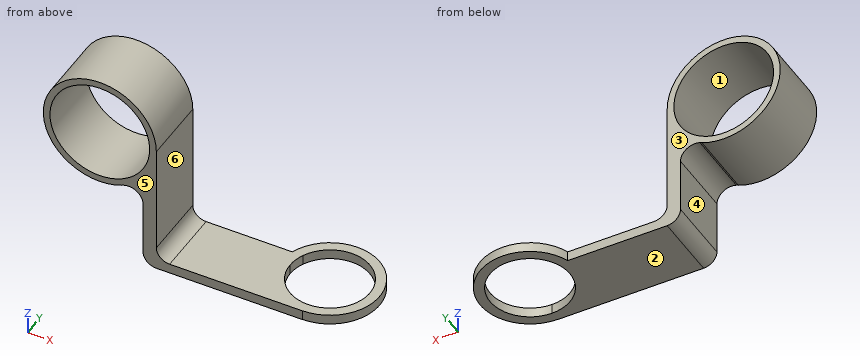
from build123d import *
from build123d.topology import SkipClean

# Parameters (mm, degrees)
SKETCH1_R           = 15
BOSS_EXTRUDE2_DEPTH = 20
CUT_EXTRUDE2_DEPTH  = 21
BOSS_EXTRUDE3_DEPTH = 3


with BuildPart() as part:
    # Sketch1 → Boss-Extrude2 (new body)
    # profile 1 of 2: a face of its own
    with BuildSketch(Plane(origin=(0, 0, 0), x_dir=(1, 0, 0), z_dir=(0, 1, 0))):
        with BuildLine():
            ThreePointArc((-50.780177481, 15.676092064), (-71.513924264, -9.412408123), (-40.357421401, 0))
            ThreePointArc((-40.357421401, 0), (-43.025497107, 9.143081868), (-50.192238582, 15.416230251))
            ThreePointArc((-50.192238582, 15.416230251), (-50.490994878, 15.535330889), (-50.780177481, 15.676092064))
        make_face()
        with Locations(Location((-57.357421401, 0, 0), (0, 0, 270))):
            Circle(SKETCH1_R, mode=Mode.SUBTRACT)
    # profile 2 of 2: a face of its own
    with BuildSketch(Plane(origin=(0, 0, 0), x_dir=(1, 0, 0), z_dir=(0, 1, 0))):
        with BuildLine():
            Line((-40.357421401, 0), (-40.357421401, 33))
            ThreePointArc((-40.357421401, 33), (-39.185848526, 35.828427125), (-36.357421401, 37))
            Line((-36.357421401, 37), (3.642578599, 37))
            Line((3.642578599, 37), (3.642578599, 40))
            Line((3.642578599, 40), (-40.357421401, 40))
            ThreePointArc((-40.357421401, 40), (-43.185848526, 38.828427125), (-44.357421401, 36))
            Line((-44.357421401, 36), (-44.357421401, 19.501688617))
            ThreePointArc((-44.357421401, 19.501688617), (-46.219952281, 15.952391985), (-50.192238582, 15.416230251))
            ThreePointArc((-50.192238582, 15.416230251), (-43.025497107, 9.143081868), (-40.357421401, 0))
        make_face()
    extrude(amount=BOSS_EXTRUDE2_DEPTH)

    # Sketch3 → Cut-Extrude2 (cut)
    with BuildSketch(Plane(origin=(0, 0, -40), x_dir=(-1, 0, 0), z_dir=(0, 0, -1))):
        with BuildLine():
            Line((-3.642578599, 20), (-3.642578599, 3))
            ThreePointArc((-3.642578599, 3), (4.842702775, 6.514718626), (8.357421401, 15))
            ThreePointArc((8.357421401, 15), (8.081425525, 17.558852734), (7.266133516, 20))
            Line((7.266133516, 20), (-3.642578599, 20))
        make_face()
        with BuildLine():
            ThreePointArc((7.266133516, 20), (-13.742083537, 21.480740698), (-3.642578599, 3))
            Line((-3.642578599, 3), (-3.642578599, 20))
            Line((-3.642578599, 20), (7.266133516, 20))
        make_face()
    extrude(amount=-CUT_EXTRUDE2_DEPTH, mode=Mode.SUBTRACT)

    # Sketch4 → Boss-Extrude3 (add)
    with SkipClean():  # the faces are left unmerged after this step: merging them gives an invalid solid
        with BuildSketch(Plane(origin=(0, 0, -40), x_dir=(-1, 0, 0), z_dir=(0, 0, -1))):
            with BuildLine():
                Line((-3.642578599, 0.051873716), (-3.642578599, 3))
                ThreePointArc((-3.642578599, 3), (-13.742083537, 21.480740698), (7.266133516, 20))
                Line((7.266133516, 20), (10.444524701, 20))
                ThreePointArc((10.444524701, 20), (-15.852965792, 23.622814157), (-3.642578599, 0.051873716))
            make_face()
        extrude(amount=-BOSS_EXTRUDE3_DEPTH)


solid = part.part
Part model, mm, in its own coordinate system. Face numbers are marked on the shaded views. A direction names the side the tool comes from. Give positions to 0.01 mm unless a question says otherwise; leave off trailing zeros. Loops run counter-clockwise (first coordinate to the right, second up) from the corner with the lowest first, then second, coordinate; pieces in that order, holes last.
(1) Pull direction Z, two halves, no side cores. Call the marked faces 1, 2 and 3: pulls with the +Z half, pulls with the -Z half, needs draft (parallel to the pull), parting line crosses it, or undercut.
Return value:
face 1: undercut
face 2: pulls with the -Z half
face 3: needs draft
(2) Band-saw the part on D-D (y = 2). Write the cut outline in (x, z), and give its area (3 significant figures).
Return value:
outline: (-50.78, -15.68) arc R4.37 cw to (-44.36, -19.5) - (-44.36, -36) arc R4 ccw to (-40.36, -40) - (11.02, -40) - (11.02, -37) - (-36.36, -37) arc R4 cw to (-40.36, -33) - (-40.36, 0) arc R17 ccw (long way) to start; hole circle Ø30 at (-57.36, 0)
area: 499 mm2
(3) Drill centre lines: line 1 along X through (y, z) = (9, -23); line 2 along Z through (x, y) = (-60, 18.25); line 3 along Z through (x, y) = (-17, 11.5). Where is each one in solid material? Low to high.
Return value:
line 1: x = -44.36 to -40.36
line 2: z = -16.79 to -14.77, 14.77 to 16.79
line 3: z = -40 to -37
(4) 3-axis set-ups, long thin cutter, end or side, ignore diameter. For the marked faces 4, 5 and 6: which of +Z, -Z, +X, -X, +Y, -Y reach the whole face in a straight line?
Return value:
face 4: -Z, -X, +Y, -Y
face 5: +Z, -Z, +X, -X, -Y
face 6: +Z, +X, +Y, -Y
(5) Band-saw the part on B-B (z = -2). Write the cut outline in (x, y), and give its area (3 significant figures).
Return value:
outline: (-74.24, 0) - (-72.22, 0) - (-72.22, 20) - (-74.24, 20) - close; (-42.49, 0) - (-40.36, 0) - (-40.36, 20) - (-42.49, 20) - close
area: 83.0 mm2
(6) Band-saw the part on C-C (x = -49). Write the cut outline in (y, z), and give its area (3 significant figures).
Return value:
outline: (0, -15.17) - (20, -15.17) - (20, -12.46) - (0, -12.46) - close; (0, 12.46) - (20, 12.46) - (20, 14.8) - (0, 14.8) - close
area: 101 mm2
(7) Band-saw the part on A-A (y = 8.25). Write the cut outline in (x, z).
Return value:
outline: (-50.78, -15.68) arc R4.37 cw to (-44.36, -19.5) - (-44.36, -36) arc R4 ccw to (-40.36, -40) - (-6.28, -40) - (-6.28, -37) - (-36.36, -37) arc R4 cw to (-40.36, -33) - (-40.36, 0) arc R17 ccw (long way) to start; (13.56, -40) - (16.98, -40) - (16.98, -37) - (13.56, -37) - close; hole circle Ø30 at (-57.36, 0)
(8) Pin check, flat tips, straight feed: pin 1 (13 mm diameter, centred on y = 13.5, z = -29.5, fed in from -X); pin 2 (10 mm diameter, centred on x = -65, y = 8.5, fed in from +Z); pin 3 (2 mm diameter, centred on y = 17.5, z = 3.5, fed in from -X). Stop position of each tip, or through.
Return value:
pin 1: stops at x = -44.36
pin 2: stops at z = 16.79
pin 3: stops at x = -74.17
